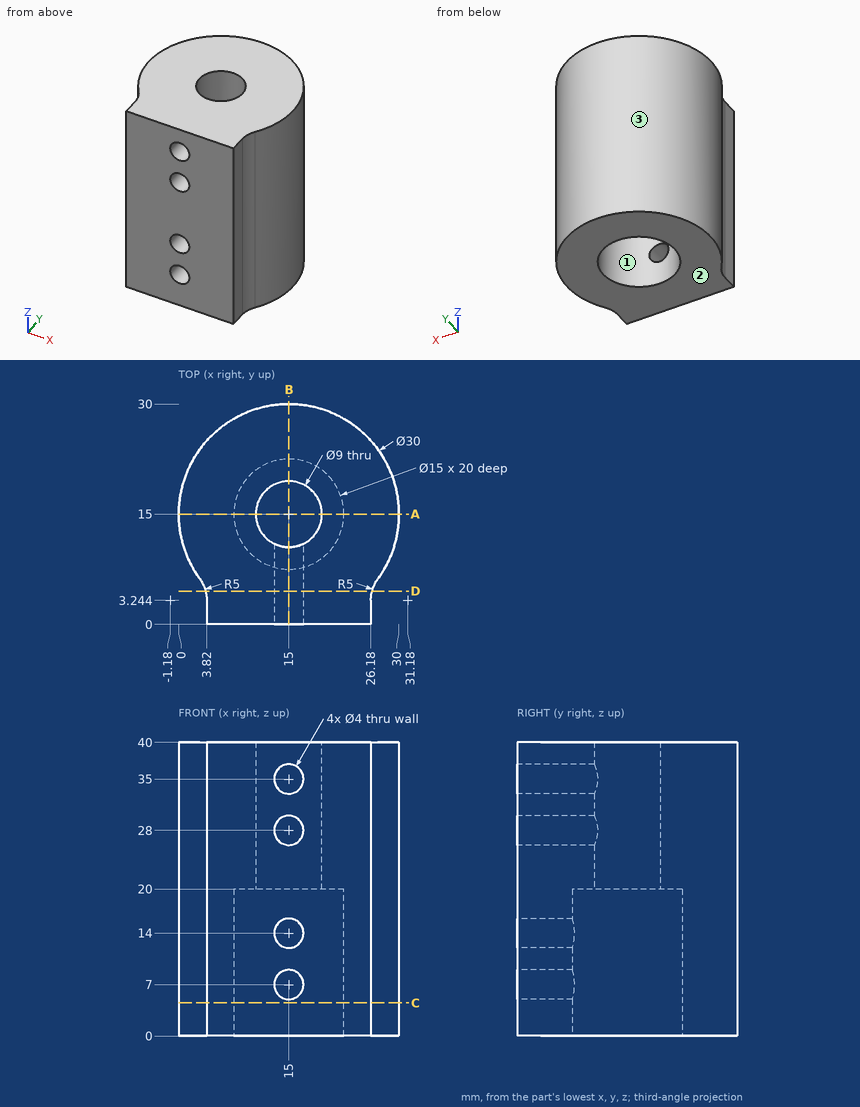
Drawing for the job (mm, zero at the part's lowest x, y, z). Give positions to 0.01 mm unless a question says otherwise; leave off trailing zeros. Loops run counter-clockwise (first coordinate to the right, second up) from the corner with the lowest first, then second, coordinate; pieces in that order, holes last.
1) Probe line 1 along Z through (x, y) = (15, 4.5); line 2 along Z through (x, y) = (15, 7.75); line 3 along Y through (x, z) = (15, 11.5). List the from-to ranges inside material, lowest first.
Values follow:
line 1: z = 0 to 5, 9 to 12, 16 to 26, 30 to 33, 37 to 40
line 2: z = 20 to 26, 30 to 33, 37 to 40
line 3: y = 0 to 7.5, 22.5 to 30
2) Band-saw the part on D-D on y = 4.5. List the corners of the cut face in (x, z), then the cut area to 3 significant figures.
Values follow:
outline: (3.66, 0) - (26.34, 0) - (26.34, 40) - (3.66, 40) - close; hole circle Ø4 at (15, 7); hole circle Ø4 at (15, 14); hole circle Ø4 at (15, 28); hole circle Ø4 at (15, 35)
area: 857 mm2
3) Band-saw the part on B-B on x = 15. List the corners of the cut face in (y, z).
Values follow:
outline: (0, 0) - (7.5, 0) - (7.5, 5) - (0, 5) - close; (0, 9) - (7.5, 9) - (7.5, 12) - (0, 12) - close; (0, 16) - (7.5, 16) - (7.5, 20) - (10.5, 20) - (10.5, 26) - (0, 26) - close; (0, 30) - (10.5, 30) - (10.5, 33) - (0, 33) - close; (0, 37) - (10.5, 37) - (10.5, 40) - (0, 40) - close; (19.5, 20) - (22.5, 20) - (22.5, 0) - (30, 0) - (30, 40) - (19.5, 40) - close
4) Band-saw the part on A-A on y = 15. List the corners of the cut face in (x, z).
Values follow:
outline: (0, 0) - (7.5, 0) - (7.5, 20) - (10.5, 20) - (10.5, 40) - (0, 40) - close; (19.5, 20) - (22.5, 20) - (22.5, 0) - (30, 0) - (30, 40) - (19.5, 40) - close
5) Two-plate mould, pull along Y, no slides. Class the marked faces 1, 2 and 3: released by +Y, released by -Y, zero draft, split by the parting line, or undercut.
Values follow:
face 1: undercut
face 2: zero draft
face 3: split by the parting line
6) Band-saw the part on C-C on z = 4.5. List the corners of the cut face in (x, y) (1 decimal).
Values follow:
outline: (2.9, 6.2) arc R5 cw to (3.8, 3.2) - (3.8, 0) - (26.2, 0) - (26.2, 3.2) arc R5 cw to (27.1, 6.2) arc R15 ccw (long way) to start; hole circle Ø15 at (15, 15)
7) Drop flat-ended pins along their axis: P1, Ø3, axis at x = 15, z = 7, coming from the -Y side; P2, Ø17, axis at x = 15, y = 15, coming from the +Z side; P3, Ø6, axis at x = 26.5, z = 17, coming from the +Y side; P4, Ø3, axis at x = 10, z = 22.5, coming from the +Y side. Give the stop position or say it passes through.
Values follow:
P1: stops at y = 22.35
P2: stops at z = 40
P3: stops at y = 27.36
P4: stops at y = 29.59
